Autodesk Fusion 360 part; units mm, degrees
sketch "Sketch1" plane through (0, 0, 0) normal (0, 1, 0) x (1, 0, 0)
  line L0 (15, -75) -> (-15, -75)
  line L1 (-15, -75) -> (-15, 75)
  line L2 (-15, 75) -> (15, 75)
  line L3 (15, 75) -> (15, -75)
  line L4 (15, -75) -> (-15, 75) construction
  line L5 (-15, -75) -> (15, 75) construction
  dimension "d1" = 150
  dimension "d2" = 30
extrude "Extrude1" add sketch "Sketch1" along normal blind 20 makes body 1
sketch "Sketch3" plane through (0, 0, -75) normal (0, 0, -1) x (1, 0, 0)
  line L0 (15, 0) -> (-15, 0)
  line L1 (-15, 0) -> (-15, -20)
  line L2 (-15, -20) -> (15, -20)
  line L3 (15, -20) -> (15, 0)
  line L4 (-15, -20) -> (15, 0)
  line L5 (15, -20) -> (-15, 0)
  circle A0 centre (0, -10) radius 70
  dimension "d5" = 140
extrude "Extrude2" add sketch "Sketch3" along normal blind 10 separate body contours L0 L4 L5 | L3 L4 L5 | L1 L4 L5 | L2 L4 L5 | A0 makes body 2
sketch "Sketch4" plane through (0, 0, 0) normal (0, -1, 0) x (1, 0, 0)
  line L0 (-15, -75) -> (15, -75)
  line L1 (15, -75) -> (15, 75)
  line L2 (15, 75) -> (-15, 75)
  line L3 (-15, 75) -> (-15, -75)
  circle A0 centre (0, 60) radius 1.6
  dimension "d8" = 3.2
  dimension "d9" = 15
  dimension "d10" = 15
extrude "Extrude3" cut sketch "Sketch4" against normal blind 35 contours A0 bodies 1
sketch "Sketch5" plane through (15, 0, 0) normal (1, 0, 0) x (0, 1, 0)
  line L0 (0, 75) -> (0, -75)
  line L1 (0, -75) -> (20, -75)
  line L2 (20, -75) -> (20, 75)
  line L3 (20, 75) -> (0, 75)
  line L4 (19.9, -65.7145) -> (-0.1, -65.7145)
  line L5 (-0.1, -65.7145) -> (-0.1, -30)
  line L6 (-0.1, -30) -> (19.9, -30)
  line L7 (19.9, -30) -> (19.9, -65.7145)
  line L8 (19.9, -65.7145) -> (-0.1, -30) construction
  line L9 (-0.1, -65.7145) -> (19.9, -30) construction
  line L10 (-60, -75) -> (80, -75)
  line L11 (-60, -85) -> (80, -85)
  line L12 (-60, -75) -> (80, -75)
  line L13 (-0.1, -65.7145) -> (0, -75)
  line L14 (19.9, -65.7145) -> (20, -75)
  line L15 (-0.1, -35) -> (19.9, -35)
  point P0 (9.9, -47.8572)
  dimension "d13" = 20
  dimension "d14" = 45
  dimension "d15" = 5
extrude "Extrude4" add sketch "Sketch5" along normal blind 48 contours L0 L6 L7 L15 bodies 1
sketch "Sketch6" plane through (0, 0, -35) normal (0, 0, -1) x (1, 0, 0)
  line L0 (15, 0) -> (15, -19.9)
  line L1 (63, -19.9) -> (63, 0)
  line L2 (63, 0) -> (15, 0)
  line L3 (58, 0) -> (63, 0)
  line L4 (63, -19.9) -> (58, -19.9)
  line L5 (63, -19.9) -> (63, 0)
  line L6 (15, -19.9) -> (63, -19.9)
  line L7 (15, -14.9) -> (58, -14.9)
  line L8 (58, -14.9) -> (58, 0)
  line L9 (58, -14.9) -> (58, -19.9)
  dimension "d18" = -5
extrude "Extrude5" add sketch "Sketch6" along normal blind 40 contours L1 L2 L3 L4 L5 L6 L8 L9 bodies 1 2
sketch "Sketch7" plane through (0, 0, 0) normal (0, -1, 0) x (1, 0, 0)
  circle A0 centre (0, 60) radius 1.6
  line L0 (15, -75) -> (15, -35)
  line L1 (15, -35) -> (58, -35)
  line L2 (58, -35) -> (58, -75)
  line L3 (63, -75) -> (63, -30)
  line L4 (63, -30) -> (15, -30)
  line L5 (15, -30) -> (15, 75)
  line L6 (15, 75) -> (-15, 75)
  line L7 (-15, 75) -> (-15, -75)
  circle A1 centre (60.5, -69.5) radius 1.6
  line L8 (-70, -75) -> (70, -75)
  circle A2 centre (11.9, -69.5) radius 1.6
  circle A3 centre (60.5, -59.6) radius 1.6
  circle A4 centre (11.9, -59.6) radius 1.6
  circle A5 centre (11.9, -39.6) radius 1.6
  circle A6 centre (11.9, -49.5) radius 1.6
  circle A7 centre (60.5, -39.6) radius 1.6
  circle A8 centre (60.5, -49.5) radius 1.6
  line L9 (-15, -75) -> (15, -75)
  line L10 (58, -75) -> (63, -75)
  dimension "d21" = 3.2
  dimension "d22" = 5.5
  dimension "d23" = 2.5
  dimension "d26" = -48.6
  dimension "d27" = 9.9
  dimension "d30" = 0
  dimension "d31" = 20
extrude "Extrude6" cut sketch "Sketch7" against normal blind 40 contours A1 | A2 | A3 | A4 | A5 | A6 | A7 | A8 bodies 1
sketch "Sketch9" plane through (0, 0, -75) normal (0, 0, 1) x (-1, 0, 0)
  line L0 (-63, 0) -> (-58, 0)
  line L1 (-58, 0) -> (-58, -19.9)
  line L2 (-58, -19.9) -> (-63, -19.9)
  line L3 (-63, -19.9) -> (-63, 0)
  circle A0 centre (0, -10) radius 70
  line L4 (15, 0) -> (15, -20)
  line L5 (15, -20) -> (-15, -20)
  line L6 (-15, -20) -> (-15, 0)
  line L7 (-15, 0) -> (15, 0)
  line L8 (-15, 0) -> (15, 0)
  circle A1 centre (21.2132, -31.2132) radius 3.25
  line L9 (0, -10) -> (21.2132, -31.2132)
  line L10 (-98.5462, -10) -> (98.5462, -10)
  circle A2 centre (21.2132, 11.2132) radius 3.25
  circle A3 centre (-21.2132, 11.2132) radius 3.25
  circle A4 centre (-21.2132, -31.2132) radius 3.25
  circle A5 centre (21.2132, -31.2132) radius 1.6
  circle A6 centre (21.2132, 11.2132) radius 1.6
  circle A7 centre (-21.2132, 11.2132) radius 1.6
  circle A8 centre (-21.2132, -31.2132) radius 1.6
  circle A9 centre (0, -10) radius 50
  circle A10 centre (-42.4264, 32.4264) radius 1.6
  line L11 (-42.4264, 32.4264) -> (0, -10)
  circle A11 centre (-42.4264, -52.4264) radius 1.6
  circle A12 centre (42.4264, -52.4264) radius 1.6
  circle A13 centre (42.4264, 32.4264) radius 1.6
  point P0 (21.2132, 11.2132)
  point P1 (-21.2132, 11.2132)
  point P2 (-21.2132, -31.2132)
  dimension "d48" = 6.5
  dimension "d53" = 30
  dimension "d54" = 45
  dimension "d56" = 360
  dimension "d57" = 3.2
  dimension "d58" = 100
  dimension "d63" = 3.2
  dimension "d64" = 60
  dimension "d65" = 45
extrude "Extrude8" cut sketch "Sketch9" against normal blind 6.5 contours A1 | A3 A7 L11 | A3 A7 L11 | A2 | A4 bodies 1
extrude "Extrude9" cut 4 faces at (-21.6042, -11.576, -75) (21.4037, -10.7748, -75) (20.8045, 30.7727, -75) (-21.4799, 30.7513, -75) along direction (0, 0, -1) blind 40 on bodies 1 bodies 1
extrude "Extrude11" cut sketch "Sketch9" against normal blind 30 contours A10 | A11 | A12 | A13 bodies 1
sketch "Sketch8" plane through (0, 0, -85) normal (0, 0, -1) x (1, 0, 0)
  circle A0 centre (21.2132, -31.2132) radius 1.6
  circle A1 centre (-21.2132, 11.2132) radius 1.6
  circle A2 centre (21.2132, 11.2132) radius 1.6
  circle A3 centre (-21.2132, -31.2132) radius 1.6
  circle A4 centre (0, -10) radius 70
  circle A5 centre (0, -10) radius 50
  circle A6 centre (0, -10) radius 11.5
  circle A7 centre (42.4264, -52.4264) radius 1.6
  circle A8 centre (42.4264, 32.4264) radius 1.6
  circle A9 centre (-42.4264, -52.4264) radius 1.6
  circle A10 centre (-42.4264, 32.4264) radius 1.6
  dimension "d59" = 100
  dimension "d60" = 23
extrude "Extrude7" cut sketch "Sketch8" against normal blind 3 contours A5 | A6 bodies 1
extrude "Extrude10" cut sketch "Sketch8" against normal blind 8.5 contours A6 bodies 1
sketch "Sketch10" plane through (0, 0, -75) normal (0, 0, 1) x (-1, 0, 0)
  circle A0 centre (-21.2132, -31.2132) radius 3.25
  circle A1 centre (-21.2132, 11.2132) radius 3.25
  circle A2 centre (21.2132, -31.2132) radius 3.25
  circle A3 centre (21.2132, 11.2132) radius 3.25
  line L0 (-63, 0) -> (-58, 0)
  line L1 (-58, 0) -> (-58, -19.9)
  line L2 (-58, -19.9) -> (-63, -19.9)
  line L3 (-63, -19.9) -> (-63, 0)
  circle A4 centre (0, -10) radius 70
  line L4 (15, 0) -> (15, -20)
  line L5 (15, -20) -> (-15, -20)
  line L6 (-15, -20) -> (-15, 0)
  line L7 (-15, 0) -> (15, 0)
  circle A5 centre (-42.4264, -52.4264) radius 1.6
  circle A6 centre (-42.4264, 32.4264) radius 1.6
  circle A7 centre (42.4264, -52.4264) radius 1.6
  circle A8 centre (42.4264, 32.4264) radius 1.6
  circle A9 centre (55, -10) radius 15
  circle A10 centre (42.4264, 32.4264) radius 1.6
  circle A11 centre (42.4264, -52.4264) radius 1.6
  circle A12 centre (-42.4264, 32.4264) radius 1.6
  circle A13 centre (-42.4264, -52.4264) radius 1.6
  circle A14 centre (0, -10) radius 70
  circle A15 centre (0, -10) radius 50
  line L8 (30.107, -14.1371) -> (66.2566, -32.5846)
  line L9 (30.107, -5.8629) -> (66.2566, 12.5846)
  point P0 (48.1818, -23.3609)
  point P1 (48.1818, 3.3609)
  dimension "d70" = 30
  dimension "d71" = 55
extrude "Extrude12" cut sketch "Sketch10" against normal blind 100 contours A4 A9 A14 L9 | A9 A15 | A4 A9 A14 L8 picked at (55.7713, -5.744) bodies 1
equation "d14 = 20 mm + 20 mm + 5 mm"
equation "d61 = -3 mm - 5.5 mm"
Read the model definition and answer for the solid it produces. Units are mm, in the model's axes. A direction names the side the tool comes from. Round coordinates to 2 decimals unless told otherwise and drop trailing zeros. Order: outer loops, then holes, each group sorted by start corner. A loop starts at its lowest first (then second) coordinate and runs counter-clockwise, first axis right, second up.
1) Flat-ended cylindrical pins translate along their axes: pin 1 (1.5 mm diameter, centred on x = -12.5, z = -18, fed in from -Y); pin 2 (1 mm diameter, centred on y = 2.5, z = 57.5, fed in from -X); pin 3 (24 mm diameter, centred on x = 1, z = 34.5, fed in from +Y). Find the tip coordinate at first contact, or state that the pin passes through.
2) For faces 1 (the face through (-15, 10, 1)), 2 (the face through (-23, 28.5, -78.2)), 3 (the face through (49.96, 12.01, -83.52)), 4 (the face through (7, 0, 1)), determine the directions among +Z, -Z, +X, -X, +Y, -Y from which every point of the face is accessible in a straight line to the end or side of a thin tool.
3) The part is cut by section A-A on z = -32.5. Write down the section's boundary in (x, y).
4) The part is cut by section B-B on x = 8. Write down the section's boundary in (y, z).
5) Straight lines are drawn through the part: L1, parallel to Z at x = 11.9, y = 12.75; L2, parallel to Y at x = 52, z = -34.5; L3, parallel to Z at x = -36, y = -41. For each, find the intervals that lie inside material, in ascending order.
6) The mould has two halves that part along X. Classify faces 5 (the face through (52, 10, -85)), 6 (the face through (-24.313, -12.189, -78.204)), 7 (the face through (63, 10, -52)): released by +X, released by -X, zero draft, split by the parting line, or undercut.
7) The part is cut by section C-C on z = 33.5. Write down the section's boundary in (x, y).
Resolved:
1. pin 1: stops at y = 0
1. pin 2: stops at x = -15
1. pin 3: stops at y = 20
2. face 1: +Z, -X, +Y, -Y
2. face 2: +Z
2. face 3: -Z
2. face 4: +Z, +X, -X, -Y
3. outline: (-15, 0) - (63, 0) - (63, 19.9) - (15, 19.9) - (15, 20) - (-15, 20) - close
4. outline: (-59.54, -85) - (-39.36, -85) - (-39.36, -82) - (1.74, -82) - (1.74, -76.5) - (18.26, -76.5) - (18.26, -82) - (59.36, -82) - (59.36, -85) - (79.54, -85) - (79.54, -75) - (20, -75) - (20, 75) - (0, 75) - (0, -75) - (-59.54, -75) - close
5. L1: z = -82 to -71.1, -67.9 to -61.2, -58 to -51.1, -47.9 to -41.2, -38 to 75
5. L2: y = 0 to 19.9
5. L3: z = -85 to -75
6. face 5: zero draft
6. face 6: undercut
6. face 7: released by +X
7. outline: (-15, 0) - (15, 0) - (15, 20) - (-15, 20) - close
